The listing builds one solid part. Answer for the finished solid, in the listing's coordinates (mm). A direction names the side the tool comes from. Coordinates: 2 decimals unless noted, no trailing zeros. Order: outer loops, then holes, each group sorted by start corner. A loop starts at its lowest first (then second) coordinate and runs counter-clockwise, first axis right, second up. Notation, with made-up numbers: (63.5, 30) -> (74.5, 30) arc R9 cw to (74.5, 47) -> close; hole circle Ø10 at (74.5, 63). An arc over 180 degrees is marked (long way). Answer in a Markdown table with one row per item.
```python
from build123d import *

# Parameters (mm, degrees)
F0_R     = 2.54
F1_DEPTH = 114.3
F2_DEPTH = 101.6
F3_DEPTH = 88.9
F4_DEPTH = 76.2
F5_DEPTH = 63.5
F6_DEPTH = 50.8
F7_DEPTH = 38.1
F8_DEPTH = 25.4
F9_DEPTH = 12.7


with BuildPart() as f1:
    # F0 (on Top) → F1 (new body)
    with BuildSketch(Plane.XY):
        Polygon((0.0297449546, -44.0977803999), (-37.9594102152, -22.2405539065), (-25.4, -43.9940905122), align=None)
        Polygon((38.0476643122, -22.0353334131), (0.0297449546, -44.0977803999), (25.2201944386, -44.2004945593), align=None)
        Polygon((-0.3350584157, 43.6933898381), (-38.2585494002, 21.7224296395), (-37.9594102152, -22.2405539065), (0.0297449546, -44.0977803999), (38.0476643122, -22.0353334131), (38.0572074327, -0.4624397172), (28.8234651499, -16.2822326428), (19.0586446504, -33.011900152), (0.0689860095, -32.9213402193), (-18.9618453465, -32.8305839378), (-28.4762239518, -16.497728885), (-38.0503063303, -0.0623833689), (-28.5255642951, 16.434953765), (-19.0890015805, 32.7795598355), (-0.3579905366, 32.7538269983), (-0.029694677, 32.9440250808), (0.3047047711, 32.7529165813), (18.8090625796, 32.7274951224), (28.6237113617, 16.568670808), (38.0578704177, 1.0362842578), (38.0671679073, 22.0539121087), align=None)
        Polygon((19.0586446504, -33.011900152), (28.8234651499, -16.2822326428), (14.47040053, -24.5877973202), (0.0689860095, -32.9213402193), align=None)
        Polygon((-18.9618453465, -32.8305839378), (0.0689860095, -32.9213402193), (-14.2417858933, -24.6875750467), (-28.4762239518, -16.497728885), align=None)
        Polygon((0.0689860095, -32.9213402193), (14.47040053, -24.5877973202), (0.1916506856, -24.6374174075), (-14.2417858933, -24.6875750467), align=None)
        Polygon((-14.2417858933, -24.6875750467), (0.1916506856, -24.6374174075), (-10.5802674086, -18.5155618092), (-21.3309908039, -12.4057515018), align=None)
        Polygon((-10.5802674086, -18.5155618092), (0.1916506856, -24.6374174075), (10.9436599796, -18.4137225871), (0.1816962855, -18.4646421982), align=None)
        Polygon((0.1916506856, -24.6374174075), (14.47040053, -24.5877973202), (21.6005177699, -12.2451052788), (10.9436599796, -18.4137225871), align=None)
        Polygon((10.9436599796, -18.4137225871), (21.6005177699, -12.2451052788), (21.5605416369, 0.4568982525), align=None)
        Polygon((10.9436599796, -18.4137225871), (21.5605416369, 0.4568982525), (10.5746748077, 18.5706432099), (-0.029694677, 18.5608677566), (18.5890194076, 0.010555068), (0.1816962855, -18.4646421982), align=None)
        Polygon((14.47040053, -24.5877973202), (28.8234651499, -16.2822326428), (28.7239362394, 0.0859907596), (21.6005177699, -12.2451052788), align=None)
        Polygon((21.6005177699, -12.2451052788), (28.7239362394, 0.0859907596), (21.5228505909, 12.4328389883), (21.5605416369, 0.4568982525), align=None)
        Polygon((38.0572074327, -0.4624397172), (38.0578704177, 1.0362842578), (28.6237113617, 16.568670808), (28.7239362394, 0.0859907596), (28.8234651499, -16.2822326428), align=None)
        Polygon((28.7239362394, 0.0859907596), (28.6237113617, 16.568670808), (14.3545600969, 24.7234572518), (21.5228505909, 12.4328389883), align=None)
        Polygon((14.3545600969, 24.7234572518), (28.6237113617, 16.568670808), (18.8090625796, 32.7274951224), (0.3047047711, 32.7529165813), align=None)
        Polygon((-28.5255642951, 16.434953765), (-0.3579905366, 32.7538269983), (-19.0890015805, 32.7795598355), align=None)
        Polygon((0.0185433098, 24.7241456127), (14.3545600969, 24.7234572518), (0.3047047711, 32.7529165813), (-0.3579905366, 32.7538269983), (-28.5255642951, 16.434953765), (-28.5009651241, 0.0160024937), (-21.37674811, 12.3222678023), (-14.1967849419, 24.7248281787), (0.0124332375, 24.7241459061), (0.0154661396, 24.7259044438), align=None)
        Polygon((-10.6340641617, 18.5510923033), (0.0124332375, 24.7241459061), (-14.1967849419, 24.7248281787), (-21.37674811, 12.3222678023), align=None)
        Polygon((-21.3540038347, 0.0308781616), (-10.6340641617, 18.5510923033), (-21.37674811, 12.3222678023), align=None)
        Polygon((-21.3540038347, 0.0308781616), (-10.5802674086, -18.5155618092), (0.1816962855, -18.4646421982), (-18.437017799, 0.0856704905), (-0.029694677, 18.5608677566), (-10.6340641617, 18.5510923033), align=None)
        Polygon((-18.437017799, 0.0856704905), (0.1816962855, -18.4646421982), (18.5890194076, 0.010555068), (-0.029694677, 18.5608677566), align=None)
        Circle(F0_R, mode=Mode.SUBTRACT)
        Circle(F0_R)
        Polygon((21.5228505909, 12.4328389883), (14.3545600969, 24.7234572518), (0.0185433098, 24.7241456127), align=None)
        Polygon((21.5228505909, 12.4328389883), (0.0185433098, 24.7241456127), (0.0124332375, 24.7241459061), (-10.6340641617, 18.5510923033), (-0.029694677, 18.5608677566), (10.5746748077, 18.5706432099), (21.5605416369, 0.4568982525), align=None)
        Polygon((-28.5009651241, 0.0160024937), (-28.5255642951, 16.434953765), (-38.0503063303, -0.0623833689), (-28.4762239518, -16.497728885), align=None)
        Polygon((-28.4762239518, -16.497728885), (-14.2417858933, -24.6875750467), (-21.3309908039, -12.4057515018), (-28.5009651241, 0.0160024937), align=None)
        Polygon((-28.5009651241, 0.0160024937), (-21.3309908039, -12.4057515018), (-21.3540038347, 0.0308781616), (-21.37674811, 12.3222678023), align=None)
        Polygon((-21.3309908039, -12.4057515018), (-10.5802674086, -18.5155618092), (-21.3540038347, 0.0308781616), align=None)
        Polygon((-37.9594102152, -22.2405539065), (-38.2585494002, 21.7224296395), (-50.8, 0), align=None)
        Polygon((50.8, 0), (38.0671679073, 22.0539121087), (38.0578704177, 1.0362842578), (38.503626573, 0.3023919341), (38.0572074327, -0.4624397172), (38.0476643122, -22.0353334131), align=None)
        Polygon((25.4, 43.9940905122), (-25.4, 43.9940905122), (-38.2585494002, 21.7224296395), (-0.3350584157, 43.6933898381), (38.0671679073, 22.0539121087), align=None)
    extrude(amount=-F1_DEPTH)

    # F0 (on Top) → F2 (cut)
    with BuildSketch(Plane.XY):
        Polygon((25.4, 43.9940905122), (-25.4, 43.9940905122), (-38.2585494002, 21.7224296395), (-0.3350584157, 43.6933898381), (38.0671679073, 22.0539121087), align=None)
        Polygon((38.0476643122, -22.0353334131), (0.0297449546, -44.0977803999), (25.2201944386, -44.2004945593), align=None)
        Polygon((0.0297449546, -44.0977803999), (-37.9594102152, -22.2405539065), (-25.4, -43.9940905122), align=None)
        Polygon((-37.9594102152, -22.2405539065), (-38.2585494002, 21.7224296395), (-50.8, 0), align=None)
        Polygon((50.8, 0), (38.0671679073, 22.0539121087), (38.0578704177, 1.0362842578), (38.503626573, 0.3023919341), (38.0572074327, -0.4624397172), (38.0476643122, -22.0353334131), align=None)
    extrude(amount=-F2_DEPTH, mode=Mode.SUBTRACT)

    # F0 (on Top) → F3 (cut)
    with BuildSketch(Plane.XY):
        Polygon((-0.3350584157, 43.6933898381), (-38.2585494002, 21.7224296395), (-37.9594102152, -22.2405539065), (0.0297449546, -44.0977803999), (38.0476643122, -22.0353334131), (38.0572074327, -0.4624397172), (28.8234651499, -16.2822326428), (19.0586446504, -33.011900152), (0.0689860095, -32.9213402193), (-18.9618453465, -32.8305839378), (-28.4762239518, -16.497728885), (-38.0503063303, -0.0623833689), (-28.5255642951, 16.434953765), (-19.0890015805, 32.7795598355), (-0.3579905366, 32.7538269983), (-0.029694677, 32.9440250808), (0.3047047711, 32.7529165813), (18.8090625796, 32.7274951224), (28.6237113617, 16.568670808), (38.0578704177, 1.0362842578), (38.0671679073, 22.0539121087), align=None)
    extrude(amount=-F3_DEPTH, mode=Mode.SUBTRACT)

    # F0 (on Top) → F4 (cut)
    with BuildSketch(Plane.XY):
        Polygon((-18.9618453465, -32.8305839378), (0.0689860095, -32.9213402193), (-14.2417858933, -24.6875750467), (-28.4762239518, -16.497728885), align=None)
        Polygon((19.0586446504, -33.011900152), (28.8234651499, -16.2822326428), (14.47040053, -24.5877973202), (0.0689860095, -32.9213402193), align=None)
        Polygon((38.0572074327, -0.4624397172), (38.0578704177, 1.0362842578), (28.6237113617, 16.568670808), (28.7239362394, 0.0859907596), (28.8234651499, -16.2822326428), align=None)
        Polygon((14.3545600969, 24.7234572518), (28.6237113617, 16.568670808), (18.8090625796, 32.7274951224), (0.3047047711, 32.7529165813), align=None)
        Polygon((-28.5255642951, 16.434953765), (-0.3579905366, 32.7538269983), (-19.0890015805, 32.7795598355), align=None)
        Polygon((-28.5009651241, 0.0160024937), (-28.5255642951, 16.434953765), (-38.0503063303, -0.0623833689), (-28.4762239518, -16.497728885), align=None)
    extrude(amount=-F4_DEPTH, mode=Mode.SUBTRACT)

    # F0 (on Top) → F5 (cut)
    with BuildSketch(Plane.XY):
        Polygon((0.0185433098, 24.7241456127), (14.3545600969, 24.7234572518), (0.3047047711, 32.7529165813), (-0.3579905366, 32.7538269983), (-28.5255642951, 16.434953765), (-28.5009651241, 0.0160024937), (-21.37674811, 12.3222678023), (-14.1967849419, 24.7248281787), (0.0124332375, 24.7241459061), (0.0154661396, 24.7259044438), align=None)
        Polygon((28.7239362394, 0.0859907596), (28.6237113617, 16.568670808), (14.3545600969, 24.7234572518), (21.5228505909, 12.4328389883), align=None)
        Polygon((14.47040053, -24.5877973202), (28.8234651499, -16.2822326428), (28.7239362394, 0.0859907596), (21.6005177699, -12.2451052788), align=None)
        Polygon((0.0689860095, -32.9213402193), (14.47040053, -24.5877973202), (0.1916506856, -24.6374174075), (-14.2417858933, -24.6875750467), align=None)
        Polygon((-28.4762239518, -16.497728885), (-14.2417858933, -24.6875750467), (-21.3309908039, -12.4057515018), (-28.5009651241, 0.0160024937), align=None)
    extrude(amount=-F5_DEPTH, mode=Mode.SUBTRACT)

    # F0 (on Top) → F6 (cut)
    with BuildSketch(Plane.XY):
        Polygon((-10.6340641617, 18.5510923033), (0.0124332375, 24.7241459061), (-14.1967849419, 24.7248281787), (-21.37674811, 12.3222678023), align=None)
        Polygon((21.5228505909, 12.4328389883), (14.3545600969, 24.7234572518), (0.0185433098, 24.7241456127), align=None)
        Polygon((-28.5009651241, 0.0160024937), (-21.3309908039, -12.4057515018), (-21.3540038347, 0.0308781616), (-21.37674811, 12.3222678023), align=None)
        Polygon((-14.2417858933, -24.6875750467), (0.1916506856, -24.6374174075), (-10.5802674086, -18.5155618092), (-21.3309908039, -12.4057515018), align=None)
        Polygon((0.1916506856, -24.6374174075), (14.47040053, -24.5877973202), (21.6005177699, -12.2451052788), (10.9436599796, -18.4137225871), align=None)
        Polygon((21.6005177699, -12.2451052788), (28.7239362394, 0.0859907596), (21.5228505909, 12.4328389883), (21.5605416369, 0.4568982525), align=None)
    extrude(amount=-F6_DEPTH, mode=Mode.SUBTRACT)

    # F0 (on Top) → F7 (cut)
    with BuildSketch(Plane.XY):
        Polygon((-21.3540038347, 0.0308781616), (-10.6340641617, 18.5510923033), (-21.37674811, 12.3222678023), align=None)
        Polygon((21.5228505909, 12.4328389883), (0.0185433098, 24.7241456127), (0.0124332375, 24.7241459061), (-10.6340641617, 18.5510923033), (-0.029694677, 18.5608677566), (10.5746748077, 18.5706432099), (21.5605416369, 0.4568982525), align=None)
        Polygon((10.9436599796, -18.4137225871), (21.6005177699, -12.2451052788), (21.5605416369, 0.4568982525), align=None)
        Polygon((-10.5802674086, -18.5155618092), (0.1916506856, -24.6374174075), (10.9436599796, -18.4137225871), (0.1816962855, -18.4646421982), align=None)
        Polygon((-21.3309908039, -12.4057515018), (-10.5802674086, -18.5155618092), (-21.3540038347, 0.0308781616), align=None)
    extrude(amount=-F7_DEPTH, mode=Mode.SUBTRACT)

    # F0 (on Top) → F8 (cut)
    with BuildSketch(Plane.XY):
        Polygon((-21.3540038347, 0.0308781616), (-10.5802674086, -18.5155618092), (0.1816962855, -18.4646421982), (-18.437017799, 0.0856704905), (-0.029694677, 18.5608677566), (-10.6340641617, 18.5510923033), align=None)
        Polygon((10.9436599796, -18.4137225871), (21.5605416369, 0.4568982525), (10.5746748077, 18.5706432099), (-0.029694677, 18.5608677566), (18.5890194076, 0.010555068), (0.1816962855, -18.4646421982), align=None)
    extrude(amount=-F8_DEPTH, mode=Mode.SUBTRACT)

    # F0 (on Top) → F9 (cut)
    with BuildSketch(Plane.XY):
        Polygon((-18.437017799, 0.0856704905), (0.1816962855, -18.4646421982), (18.5890194076, 0.010555068), (-0.029694677, 18.5608677566), align=None)
        Circle(F0_R, mode=Mode.SUBTRACT)
    extrude(amount=-F9_DEPTH, mode=Mode.SUBTRACT)


solid = f1.part
```
(1) Which of the six approach directions +Z, -Z, +X, -X, +Y, -Y give full straight-line access (tool end or side, diameter ignored) to faces 1 (the flat face through (-15, -28, -76.2)), 2 (the flat face through (43, 0, -101.6)), 3 (the flat face through (15, -4, -25.4)), 4 (the flat face through (-17, 9, -38.1))?
Check values:
| item | result |
|---|---|
| face 1 | +Z, -X, -Y |
| face 2 | +Z, +X, +Y, -Y |
| face 3 | +Z, +X |
| face 4 | +Z, -X, +Y |
(2) A cutting plane is placed at C-C, the plane x = 36. Determine the outline of the cut face in (y, z), then the cut area to 3 significant figures.
Check values:
| item | result |
|---|---|
| outline | (-25.57, -114.3) -> (25.63, -114.3) -> (25.63, -101.6) -> (23.22, -101.6) -> (23.22, -88.9) -> (4.42, -88.9) -> (4.42, -76.2) -> (-3.99, -76.2) -> (-3.99, -88.9) -> (-23.22, -88.9) -> (-23.22, -101.6) -> (-25.57, -101.6) -> close |
| area | 1,350 mm² |
(3) Find the intervals of material crossed by line 1 along Y through (x, z) = (-20.5, -103.5); line 2 along Z through (x, y) = (-11.5, -32); line 3 along Z through (x, y) = (20, 2), in increasing order. Write a range as from..to.
Check values:
| item | result |
|---|---|
| line 1 | -44.01..43.99 |
| line 2 | -114.3..-76.2 |
| line 3 | -114.3..-25.4 |
(4) Flat-ended cylindrical pins translate along their axes: pin 1 (6.5 mm diameter, centred on x = 11.5, y = 0.5, fed in from +Z); pin 2 (10 mm diameter, centred on y = -21.5, z = -29.5, fed in from +X); pin 3 (18 mm diameter, centred on x = -14, y = -20.5, fed in from +Z). Find the tip coordinate at first contact, or state that the pin passes through.
Check values:
| item | result |
|---|---|
| pin 1 | z = -12.7 |
| pin 2 | x = 12.02 |
| pin 3 | z = -25.4 |
(5) A cutting plane is placed at D-D, the plane z = -54. Determine the outline of the cut face in (x, y).
Check values:
| item | result |
|---|---|
| outline | (-28.5, 0.02) -> (-14.24, -24.69) -> (14.47, -24.59) -> (28.72, 0.09) -> (14.35, 24.72) -> (-14.2, 24.72) -> close |
